Autodesk Inventor part; units mm, degrees
ref_plane "YZ Plane" through (0, 0, 0) normal (1, 0, 0) x (0, 1, 0)
ref_plane "XZ Plane" through (0, 0, 0) normal (0, 1, 0) x (-1, 0, 0)
ref_plane "XY Plane" through (0, 0, 0) normal (0, 0, 1) x (1, 0, 0)
sketch "Sketch1" plane through (0, 0, 0) normal (0, 0, 1) x (1, 0, 0)
  line L0 (0, 0) -> (19.939, 0)
  line L1 (19.939, 0) -> (19.939, 25.4)
  line L2 (19.939, 25.4) -> (0, 25.4)
  line L3 (0, 25.4) -> (0, 0)
  dimension "d0" = 19.939
  dimension "d1" = 25.4
extrude "Extrusion1" add sketch "Sketch1" along normal blind 25.4
shell "Shell1" thickness 2.54 removed faces 1 at (13.2927, 25.4, 8.4667)
sketch "Sketch2" plane through (0, 0, 25.4) normal (0, 0, 1) x (1, 0, 0)
  line L0 (15.367, 1.905) -> (4.572, 1.905)
  line L1 (4.572, 1.905) -> (4.572, 17.145)
  line L2 (4.572, 17.145) -> (15.367, 17.145)
  line L3 (15.367, 17.145) -> (15.367, 1.905)
  line L4 (15.367, 1.905) -> (4.572, 17.145) construction
  line L5 (4.572, 1.905) -> (15.367, 17.145) construction
  line L6 (0, 25.4) -> (0, 0)
  line L7 (0, 0) -> (19.939, 0)
  circle A0 centre (9.9695, 6.985) radius 3.175
  circle A1 centre (6.7945, 14.9098) radius 1.5875
  circle A2 centre (13.1318, 14.9098) radius 1.5875
  line L8 (19.939, 0) -> (19.939, 25.4)
  point P0 (9.9695, 9.525)
  dimension "d5" = 9.9695
  dimension "d6" = 9.525
  dimension "d7" = 15.24
  dimension "d8" = 10.795
  dimension "d9" = 6.35
  dimension "d10" = 5.08
  dimension "d11" = 3.175
  dimension "d12" = 7.9248
  dimension "d13" = 3.175
  dimension "d15" = 6.7945
  dimension "d16" = 6.8072
  dimension "d24" = 6.985
hole "Hole1" at (13.1318, 14.9098, 25.4) at (6.7945, 14.9098, 25.4) direction (0, 0, -1) diameter 3.175 depth 7.62 tip angle 118
sketch "Sketch3" plane through (0, 0, 25.4) normal (0, 0, 1) x (1, 0, 0)
  circle A0 centre (9.9695, 6.985) radius 6.35
  line L0 (0, 0) -> (19.939, 0)
  line L1 (19.939, 0) -> (19.939, 25.4)
  dimension "d25" = 12.7
  dimension "d26" = 6.985
  dimension "d27" = 9.9695
hole "Hole2" at (9.9695, 6.985, 25.4) direction (0, 0, -1) diameter 12.7 depth 2.54 tip angle 118
sketch "Sketch4" plane through (0, 0, 25.4) normal (0, 0, 1) x (1, 0, 0)
  line L0 (17.1577, 1.905) -> (2.8067, 1.905)
  line L1 (2.8067, 1.905) -> (2.8067, 17.145)
  line L2 (2.8067, 17.145) -> (17.1577, 17.145)
  line L3 (17.1577, 17.145) -> (17.1577, 1.905)
  line L4 (17.1577, 1.905) -> (2.8067, 17.145) construction
  line L5 (2.8067, 1.905) -> (17.1577, 17.145) construction
  line L6 (0, 0) -> (19.939, 0)
  line L7 (0, 25.4) -> (0, 0)
  circle A0 centre (13.1318, 14.9352) radius 1.5875
  circle A1 centre (6.7945, 14.9352) radius 1.5875
  line L8 (19.939, 0) -> (19.939, 25.4)
  circle A2 centre (9.9695, 6.985) radius 6.35
  point P0 (9.9822, 9.525)
  dimension "d35" = 9.525
  dimension "d36" = 14.351
  dimension "d38" = 9.9822
  dimension "d39" = 6.8072
  dimension "d40" = 6.7945
  dimension "d41" = 12.7
  dimension "d42" = 9.9695
  dimension "d43" = 5.08
  dimension "d44" = 7.9502
  dimension "d45" = 7.9502
  dimension "d56" = 6.3373
  dimension "d66" = 1.905
  dimension "d75" = 2.8067
  dimension "d76" = 2.7813
sketch "Sketch5" plane through (0, 0, 25.4) normal (0, 0, 1) x (1, 0, 0)
  point P0 (0, 0)
extrude "Extrusion2" add sketch "Sketch4" along normal blind 4.7625 contours L0 A2 L1 L2 L3
sketch "Sketch6" plane through (0, 0, 30.1625) normal (0, 0, 1) x (1, 0, 0)
  line L0 (17.1577, 1.905) -> (2.8067, 1.905)
  line L1 (8.6487, 1.905) -> (11.3157, 1.905)
  line L2 (11.3157, 1.905) -> (11.3157, 40.005)
  line L3 (11.3157, 40.005) -> (8.6487, 40.005)
  line L4 (8.6487, 40.005) -> (8.6487, 1.905)
  line L5 (17.1577, 1.905) -> (17.1577, 17.145)
  point P0 (0, 0)
  dimension "d48" = 2.667
  dimension "d49" = 5.842
  dimension "d71" = 38.1
extrude "Extrusion3" cut sketch "Sketch6" against normal blind 3.175
sketch "Sketch9" plane through (2.54, 2.54, 2.54) normal (0, 0, 1) x (1, 0, 0)
  line L0 (1.8542, 12.7) -> (6.9342, 12.7)
  line L1 (6.9342, 12.7) -> (6.9342, 7.9375)
  line L2 (6.9342, 7.9375) -> (1.8542, 7.9375)
  line L3 (1.8542, 7.9375) -> (1.8542, 12.7)
  line L4 (7.9375, 12.7) -> (14.2875, 12.7)
  line L5 (14.2875, 12.7) -> (14.2875, 7.9375)
  line L6 (14.2875, 7.9375) -> (7.9375, 7.9375)
  line L7 (7.9375, 7.9375) -> (7.9375, 12.7)
  line L8 (0, 22.86) -> (14.859, 22.86)
  line L9 (0, 22.86) -> (0, 0)
  point P0 (-2.54, -2.54)
  dimension "d97" = 10.16
  dimension "d98" = 5.08
  dimension "d100" = 1.8542
  dimension "d101" = 4.7625
extrude "Extrusion5" add sketch "Sketch9" along normal blind 5.08 contours L0 L1 L2 L3
sketch "Sketch10" plane through (2.54, 2.54, 2.54) normal (0, 0, 1) x (1, 0, 0)
  line L0 (7.9375, 7.9375) -> (13.0175, 7.9375)
  line L1 (13.0175, 7.9375) -> (13.0175, 12.7)
  line L2 (13.0175, 12.7) -> (7.9375, 12.7)
  line L3 (7.9375, 12.7) -> (7.9375, 7.9375)
  line L4 (0, 22.86) -> (14.859, 22.86)
  line L5 (1.8542, 12.7) -> (6.9342, 12.7)
  point P0 (-2.54, -2.54)
  dimension "d94" = 5.08
  dimension "d95" = 10.16
  dimension "d96" = 10.16
  dimension "d99" = 1.8415
  dimension "d102" = 4.7625
extrude "Extrusion6" add sketch "Sketch10" along normal blind 5.08
sketch "Sketch11" plane through (0, 0, 0) normal (0, 0, -1) x (-1, 0, 0)
  circle A0 centre (-13.1445, 12.7) radius 1.5875
  circle A1 centre (-6.7945, 12.7) radius 1.5875
  line L0 (0, 25.4) -> (0, 0)
  line L1 (-19.939, 0) -> (-19.939, 25.4)
  line L2 (0, 0) -> (-19.939, 0)
  dimension "d81" = 6.7945
  dimension "d91" = 12.7
  dimension "d92" = 12.7
  dimension "d93" = 6.35
hole "Hole4" at (13.1445, 12.7, 0) at (6.7945, 12.7, 0) direction (0, 0, 1) diameter 3.175 depth 15.24 tip angle 118
sketch "Sketch12" plane through (0, 25.4, 0) normal (0, 1, 0) x (1, 0, 0)
  line L0 (0, 0) -> (0, -25.4)
  line L1 (19.939, 0) -> (19.939, -25.4)
  line L2 (0, 0) -> (19.939, 0)
  line L3 (19.939, 0) -> (19.939, -25.4)
  line L4 (19.939, -25.4) -> (0, -25.4)
  line L5 (0, -25.4) -> (0, 0)
extrude "Extrusion7" add sketch "Sketch12" along normal blind 18.1429
sketch "Sketch13" plane through (0, 43.5429, 0) normal (0, 1, 0) x (1, 0, 0)
  line L0 (2.54, -2.54) -> (17.399, -2.54)
  line L1 (17.399, -2.54) -> (17.399, -25.4)
  line L2 (17.399, -25.4) -> (2.54, -25.4)
  line L3 (2.54, -25.4) -> (2.54, -2.54)
  line L4 (19.939, 0) -> (0, 0)
  line L5 (0, 0) -> (0, -25.4)
  line L6 (19.939, -25.4) -> (19.939, 0)
  dimension "d105" = 2.54
  dimension "d106" = 2.54
  dimension "d107" = 25.4
  dimension "d110" = 2.54
extrude "Extrusion8" cut sketch "Sketch13" against normal blind 18.1429
sketch "Sketch14" plane through (0, 0, 25.4) normal (0, 0, 1) x (1, 0, 0)
  line L0 (2.8067, 36.5125) -> (17.1577, 36.5125)
  line L1 (17.1577, 36.5125) -> (17.1577, 31.75)
  line L2 (17.1577, 31.75) -> (2.8067, 31.75)
  line L3 (2.8067, 31.75) -> (2.8067, 36.5125)
  line L4 (0, 0) -> (0, 43.5429)
  line L5 (19.939, 0) -> (19.939, 43.5429)
  line L6 (2.8067, 17.145) -> (2.8067, 1.905)
  line L7 (17.1577, 1.905) -> (17.1577, 17.145)
  dimension "d134" = 0
  dimension "d135" = 0
extrude "Extrusion9" add sketch "Sketch14" along normal blind 4.7625 and the other way blind 2.54
sketch "Sketch15" plane through (0, 0, 30.1625) normal (0, 0, 1) x (1, 0, 0)
  line L0 (2.8067, 31.75) -> (17.1577, 31.75)
  line L1 (8.6487, 31.75) -> (11.3157, 31.75)
  line L2 (11.3157, 31.75) -> (11.3157, 36.5125)
  line L3 (11.3157, 36.5125) -> (8.6487, 36.5125)
  line L4 (8.6487, 36.5125) -> (8.6487, 31.75)
  line L5 (2.8067, 36.5125) -> (2.8067, 31.75)
  line L6 (17.1577, 31.75) -> (17.1577, 36.5125)
  line L7 (17.1577, 36.5125) -> (2.8067, 36.5125)
  line L8 (19.939, 0) -> (19.939, 43.5429)
  line L9 (17.399, 43.5429) -> (17.399, 25.4)
  line L10 (17.1577, 1.905) -> (17.1577, 17.145)
  point P0 (0, 0)
  point P1 (17.399, 31.75)
  dimension "d119" = 0
  dimension "d130" = 2.667
  dimension "d133" = 5.842
extrude "Extrusion10" cut sketch "Sketch15" against normal blind 3.175 contours L4 L3 L2 L0
sketch "Sketch16" plane through (0, 0, 30.1625) normal (0, 0, 1) x (1, 0, 0)
  circle A0 centre (6.8072, 34.0179) radius 1.5875
  circle A1 centre (13.1318, 34.0179) radius 1.5875
  line L0 (0, 0) -> (0, 43.5429)
  line L1 (19.939, 0) -> (19.939, 43.5429)
  line L2 (2.54, 43.5429) -> (17.399, 43.5429)
  dimension "d122" = 3.175
  dimension "d123" = 3.175
  dimension "d124" = 6.8072
  dimension "d125" = 6.8072
  dimension "d126" = 9.525
  dimension "d127" = 9.525
extrude "Extrusion11" cut sketch "Sketch16" against normal blind 12.7
sketch "Sketch17" plane through (0, 0, 25.4) normal (0, 0, 1) x (1, 0, 0)
  line L0 (17.1577, 36.5125) -> (17.1577, 31.75)
  line L1 (19.939, 0) -> (19.939, 43.5429)
  line L2 (17.1577, 31.75) -> (19.939, 31.75)
  line L3 (19.939, 31.75) -> (19.939, 36.5125)
  line L4 (19.939, 36.5125) -> (17.1577, 36.5125)
  line L5 (17.1577, 36.5125) -> (17.1577, 31.75)
  line L6 (2.8067, 31.75) -> (2.8067, 36.5125)
  line L7 (0, 0) -> (0, 43.5429)
  line L8 (2.8067, 31.75) -> (0, 31.75)
  line L9 (0, 31.75) -> (0, 36.5125)
  line L10 (0, 36.5125) -> (2.8067, 36.5125)
  line L11 (2.8067, 36.5125) -> (2.8067, 31.75)
extrude "Extrusion12" add sketch "Sketch17" against normal blind 2.54
equation "\"d125\" = d124"
equation "\"d127\" = d126"
properties part number "BasePlateBottom"
Check sheet for the modelled part. Datum: model origin and axes. Units: mm. A direction names the side the tool comes from. Round coordinates to 2 decimals unless told otherwise and drop trailing zeros. Loops run counter-clockwise (first coordinate to the right, second up) from the corner with the lowest first, then second, coordinate; pieces in that order, holes last. Notation, with made-up numbers: (75, 89) -> (116, 89) arc R15 cw to (116, 110) -> close; hole circle Ø3 at (84, 20.5). An arc over 180 degrees is marked (long way). Answer in a Markdown table with one row per item.
Q1. Set-up check for faces 4 (the face through (10.1, 36.512, 26.6)), 5 (the face through (17.158, 10, 28)), 6 (the face through (5, 1.905, 28)), 7 (the face through (11.316, 34, 29)): record each of +Z, -Z, +X, -X, +Y, -Y from which the full face is reachable in a straight line by a thin tool's end or side.
Data:
| item | result |
|---|---|
| face 4 | +Z, +Y |
| face 5 | +Z, +X, +Y, -Y |
| face 6 | +Z, +X, -X, -Y |
| face 7 | +Z, +Y, -Y |
Q2. Sectioned sample at C-C on y = 27.5. Enter the section's corners in (x, z).
Data:
| item | result |
|---|---|
| outline | (0, 0) -> (19.94, 0) -> (19.94, 25.4) -> (17.4, 25.4) -> (17.4, 2.54) -> (2.54, 2.54) -> (2.54, 25.4) -> (0, 25.4) -> close |
Q3. Release check for a two-part mould opening along Y. For faces 1 (the face through (17.158, 34, 28)), 2 (the face through (10, 0, 13)), 3 (the face through (6.46, 32.47, 26.56)) record: released by +Y, released by -Y, zero draft, split by the parting line, or undercut.
Data:
| item | result |
|---|---|
| face 1 | zero draft |
| face 2 | released by -Y |
| face 3 | undercut |
Q4. Sectioned sample at D-D on z = 21. Enter the section's corners in (x, y).
Data:
| item | result |
|---|---|
| outline | (0, 0) -> (19.94, 0) -> (19.94, 43.54) -> (17.4, 43.54) -> (17.4, 2.54) -> (2.54, 2.54) -> (2.54, 43.54) -> (0, 43.54) -> close |
Q5. Sectioned sample at B-B on y = 12.7. Give the number of separate pieces and of enclosed holes in the cut face, then the cut area to 3 significant figures.
Data:
| item | result |
|---|---|
| separate pieces | 3 |
| enclosed holes | 0 |
| area | 236 mm^2 |
Q6. Go/stop test with flat-tipped pins: P1, Ø3.5, axis at x = 4.5, z = 28.5, coming from the -Y side (3 decimals); P2, Ø0.8, axis at x = 10, y = 35.5, coming from the +Z side; P3, Ø2.5, axis at x = 7, z = 4.5, coming from the +Y side. Record where each tip stops, or that it passes through.
Data:
| item | result |
|---|---|
| P1 | stops at y = 1.905 |
| P2 | stops at z = 26.99 |
| P3 | stops at y = 15.24 |
Q7. Sectioned sample at A-A on z = 3.5. Enter the section's corners in (x, y) (1 decimal), then the cut area to 3 significant figures.
Data:
| item | result |
|---|---|
| outline | (0, 0) -> (19.9, 0) -> (19.9, 43.5) -> (17.4, 43.5) -> (17.4, 2.5) -> (2.5, 2.5) -> (2.5, 43.5) -> (0, 43.5) -> close; (4.4, 10.5) -> (9.5, 10.5) -> (9.5, 15.2) -> (4.4, 15.2) -> close; (10.5, 10.5) -> (15.6, 10.5) -> (15.6, 15.2) -> (10.5, 15.2) -> close; hole circle Ø3.2 at (6.8, 12.7); hole circle Ø3.2 at (13.1, 12.7) |
| area | 291 mm^2 |
Q8. Thickness scan on L1, parallel to X at y = 16.5, z = 18.5; L2, parallel to X at y = 12, z = 4; L3, parallel to Z at x = 4.5, y = 20.5. Record the ranges inside material, lowest first.
Data:
| item | result |
|---|---|
| L1 | x = 0 to 2.54, 17.4 to 19.94 |
| L2 | x = 0 to 2.54, 4.39 to 5.37, 8.22 to 9.47, 10.48 to 11.72, 14.57 to 15.56, 17.4 to 19.94 |
| L3 | z = 0 to 2.54, 22.86 to 25.4 |
